Autodesk Inventor part; units mm, degrees
ref_plane "YZ Plane" through (0, 0, 0) normal (1, 0, 0) x (0, 1, 0)
ref_plane "XZ Plane" through (0, 0, 0) normal (0, 1, 0) x (-1, 0, 0)
ref_plane "XY Plane" through (0, 0, 0) normal (0, 0, 1) x (1, 0, 0)
sketch "Sketch1" plane through (0, 0, 0) normal (0, 1, 0) x (-1, 0, 0)
  circle A0 centre (0, 0) radius 1.5
  dimension "d0" = 3
extrude "Extrusion1" add sketch "Sketch1" along normal blind 10
sketch "Sketch2" plane through (0, 0, 0) normal (0, -1, 0) x (1, 0, 0)
  line L0 (6, 5) -> (-6, 5)
  line L1 (-6, 5) -> (-6, -5)
  line L2 (-6, -5) -> (6, -5)
  line L3 (6, -5) -> (6, 5)
  line L4 (6, 5) -> (-6, -5) construction
  line L5 (-6, 5) -> (6, -5) construction
  point P0 (0, 0)
  point P1 (0, 0)
  point P2 (0, 0)
  point P3 (0, 0)
  dimension "d3" = 10
  dimension "d4" = 12
extrude "Extrusion2" add sketch "Sketch2" along normal blind 9
sketch "Sketch3" plane through (6, 0, 5) normal (1, 0, 0) x (0, 0, -1)
  line L0 (10, 0) -> (0, 0)
  line L1 (0, 0) -> (0, -9)
  line L2 (10, -9) -> (0, -9)
  line L3 (10, 0) -> (10, -9)
  line L4 (0, 0) -> (0, -9)
  line L5 (0, -4.5) -> (10, -4.5)
  line L6 (10, 0) -> (10, -9)
  point P0 (5, 0)
  point P1 (0, -4.5)
extrude "Extrusion3" add sketch "Sketch3" along normal blind 12 contours L3 L2 L1 L5
sketch "Sketch4" plane through (6, -4.5, 5) normal (0, 1, 0) x (1, 0, 0)
  line L0 (0, 0) -> (0, 10)
  line L1 (0, 0) -> (12, 0)
  line L2 (12, 10) -> (12, 0)
  line L3 (0, 10) -> (12, 10)
  circle A0 centre (6, 5) radius 5
  point P0 (-6, 5)
  point P1 (12, 5)
  point P2 (6, 0)
  dimension "d9" = 10
extrude "Extrusion4" add sketch "Sketch4" along normal blind 10.5 contours A0
fillet "Fillet1" radius 1 4 edges at (-6, -4.5, 5) (18, -6.75, 5) (18, -6.75, -5) (-6, -4.5, -5)
sketch "Sketch5" plane through (0, 10, 0) normal (0, 1, 0) x (1, 0, 0)
  circle A0 centre (0, 0) radius 1.5
  line L0 (-1, -1.118) -> (-1, 1.118)
  circle A1 centre (0, 0) radius 1.5
  dimension "d13" = 0.5
extrude "Extrusion5" cut sketch "Sketch5" against normal blind 9 contours L0 A0 picked at (-1.1631, -0.0599)
properties part number "GM1024BY10" material "Bronze, Soft Tin"
Work out the finished part from the listing and answer in its coordinate system (mm). A direction names the side the tool comes from. Give positions to 0.01 mm unless a question says otherwise; leave off trailing zeros. Loops run counter-clockwise (first coordinate to the right, second up) from the corner with the lowest first, then second, coordinate; pieces in that order, holes last. Notation, with made-up numbers: (60.5, 83.5) -> (69.5, 83.5) arc R29 ccw to (69.5, 113.5) -> close; hole circle Ø11 at (21, 24.25). An arc over 180 degrees is marked (long way). Put each result on its own line as item: value. Start each with the question number.
Item 1: The part is cut by section A-A (x = 15). Give the vertices of the cut face in (y, z), then the cut area to 3 significant figures.
Item 2: Each of these flat-tipped pins is pushed along its axis until it touches: P1, Ø1, axis at x = 15, z = 2, coming from the +Y side; P2, Ø5, axis at y = -1, z = -0.5, coming from the +X side; P3, Ø1, axis at x = 8, y = 5, coming from the +Z side. Where does it stop, or does it pass through?
Item 3: The part is cut by section C-C (x = 0). Give the vertices of the cut face in (y, z).
Item 4: The part is cut by section B-B (z = 0). Give the vertices of the cut face in (x, y), then the cut area to 4 significant figures.
Item 5: The part is cut by section D-D (z = -2). Give the vertices of the cut face in (x, y).
Item 6: The mould has two halves that part along X. Classify faces 1 (the face through (-5.699, -4.563, 4.715)), 2 (the face through (1.2, 0, 1.2)), 3 (the face through (12, 6, 0)), 4 (the face through (1.5, 4.93, -0.07)): released by +X, released by -X, zero draft, split by the parting line, or undercut.
Item 7: Which of the six approach directions +Z, -Z, +X, -X, +Y, -Y give full straight-line access (tool end or side, diameter ignored) to faces 5 (the face through (-1, 6, 0)), 6 (the face through (17.2, -4.5, -0.3)), 7 (the face through (16.77, 0.68, 1.5)), 8 (the face through (6, -2, 0))?
Item 8: Find the intervals of material crossed by L1, parallel to Y at x = 10, z = 3; L2, parallel to Y at x = -2, z = 1.5; L3, parallel to X at y = 4.5, z = 0, in increasing order. Write a range as [from, to].
Answers below:
1. outline: (-9, -5) -> (-4.5, -5) -> (-4.5, -4) -> (6, -4) -> (6, 4) -> (-4.5, 4) -> (-4.5, 5) -> (-9, 5) -> close
1. area: 129 mm2
2. P1: y = 6
2. P2: x = 17
2. P3: z = 3.57
3. outline: (-9, -5) -> (0, -5) -> (0, -1.5) -> (10, -1.5) -> (10, 1.5) -> (0, 1.5) -> (0, 5) -> (-9, 5) -> close
4. outline: (-6, -9) -> (18, -9) -> (18, -4.5) -> (17, -4.5) -> (17, 6) -> (7, 6) -> (7, -4.5) -> (6, -4.5) -> (6, 0) -> (1.5, 0) -> (1.5, 10) -> (-1, 10) -> (-1, 1) -> (-1.5, 1) -> (-1.5, 0) -> (-6, 0) -> close
4. area: 292.5 mm2
5. outline: (-6, -9) -> (18, -9) -> (18, -4.5) -> (16.58, -4.5) -> (16.58, 6) -> (7.42, 6) -> (7.42, -4.5) -> (6, -4.5) -> (6, 0) -> (-6, 0) -> close
6. face 1: released by -X
6. face 2: undercut
6. face 3: zero draft
6. face 4: undercut
7. face 5: +Z, -Z, -X, +Y
7. face 6: +X, +Y
7. face 7: +Y
7. face 8: +Z, -Z, +Y
8. L1: [-9, 6]
8. L2: [-9, 0]
8. L3: [-1, 1.5], [7, 17]
